Verification items for the finished model (mm, model axes). A direction names the side the tool comes from. Give positions to 0.01 mm unless a question says otherwise; leave off trailing zeros. Loops run counter-clockwise (first coordinate to the right, second up) from the corner with the lowest first, then second, coordinate; pieces in that order, holes last. Notation, with made-up numbers: M 4,-24.5 L 29,-24.5 A27 ccw 29,0.5 Z; hole C -19,31 d8. An arc over 180 degrees is marked long. Put each result on its own line as item: value. Start each with the question number.
from build123d import *

# Parameters (mm, degrees)
F0_W     = 200
F0_H     = 250
F1_DEPTH = 25
F2_W     = 80
F2_H     = 250
F3_DEPTH = 50
F4_R     = 37.5
F5_DEPTH = 137


with BuildPart() as f1:
    # F0 (on Top) → F1 (new body, symmetric)
    with BuildSketch(Plane.XY):
        Rectangle(F0_W, F0_H)
    extrude(amount=F1_DEPTH, both=True)

    # F2 (on face) → F3 (join)
    with BuildSketch(Plane.XY.offset(25)):
        Rectangle(F2_W, F2_H)
    extrude(amount=F3_DEPTH)

    # F4 (on face) → F5 (cut)
    with BuildSketch(Plane.XY.offset(75)):
        Circle(F4_R)
    extrude(amount=-F5_DEPTH, mode=Mode.SUBTRACT)


solid = f1.part
Q1. Cross-section at A-A, the plane y = 0. Record the boundary of the cut face in (x, z).
Q2. Cross-section at C-C, the plane z = 36. Record the boundary of the cut face in (x, y).
Q3. Cross-section at B-B, the plane x = 0. Record the boundary of the cut face in (y, z).
Q4. Set-up check for faces 1 (the face through (70, 2, 25)), 2 (the face through (-24, 30, -25)), 3 (the face through (-40, -2, 50)): record each of +Z, -Z, +X, -X, +Y, -Y from which the full face is reachable in a straight line by a thin tool's end or side.
Q5. Scan lines: L1, parallel to Y at x = 0, z = 41; L2, parallel to Z at x = -61, y = 20; L3, parallel to X at y = 109, z = 32.5. Record each from-to range of solid material in increasing order.
Q6. Go/stop test with flat-tipped pins: pin 1 (1.5 mm diameter, centred on y = -18.5, z = 61, fed in from +X); pin 2 (8 mm diameter, centred on x = -3.5, y = 32.5, fed in from -Z). Record where each tip stops, or that it passes through.
Q7. Release check for a two-part mould opening along Y. For faces 4 (the face through (-1, -125, 15)), 5 (the face through (-4.88, 37.18, 25.7)), 6 (the face through (-1, 125, 15)), 7 (the face through (-27, 30, 75)) record: pulls with the +Y half, pulls with the -Y half, needs draft (parallel to the pull), parting line crosses it, or undercut.
Q8. Cross-section at D-D, the plane y = -87. Record the boundary of the cut face in (x, z).
Ans:
1. outline: M -100,-25 L -37.5,-25 L -37.5,75 L -40,75 L -40,25 L -100,25 Z; M 37.5,-25 L 100,-25 L 100,25 L 40,25 L 40,75 L 37.5,75 Z
2. outline: M -40,-125 L 40,-125 L 40,125 L -40,125 Z; hole C 0,0 d75
3. outline: M -125,-25 L -37.5,-25 L -37.5,75 L -125,75 Z; M 37.5,-25 L 125,-25 L 125,75 L 37.5,75 Z
4. face 1: +Z, +X, +Y, -Y
4. face 2: -Z, +X, -X, +Y, -Y
4. face 3: +Z, -X, +Y, -Y
5. L1: y = -125 to -37.5, 37.5 to 125
5. L2: z = -25 to 25
5. L3: x = -40 to 40
6. pin 1: stops at x = 40
6. pin 2: passes through
7. face 4: pulls with the -Y half
7. face 5: undercut
7. face 6: pulls with the +Y half
7. face 7: needs draft
8. outline: M -100,-25 L 100,-25 L 100,25 L 40,25 L 40,75 L -40,75 L -40,25 L -100,25 Z
